Here's how the part is built. I have some questions about the finished solid (model axes, mm). A direction names the side the tool comes from. Give positions to 0.01 mm unless a question says otherwise; leave off trailing zeros. Loops run counter-clockwise (first coordinate to the right, second up) from the corner with the lowest first, then second, coordinate; pieces in that order, holes last. Notation, with made-up numbers: (68, 35) - (117, 35) arc R27 ccw to (117, 66) - close; hole circle Ø3 at (2.5, 77). An arc over 180 degrees is marked (long way). One line per item, written item: value. Start each with the question number.
```python
from build123d import *

# Parameters (mm, degrees)
F1_DEPTH = 2.54
F2_SIZE  = 2.53999
F4_DEPTH = 2.54
F5_SIZE  = 2.032


# Not quite as in the source:
# - a fillet or chamfer is up to 0.001 mm smaller than in the source, because OpenCascade refuses the exact size


with BuildPart() as f1:
    # F0 (on Top) → F1 (new body, symmetric)
    with BuildSketch(Plane.XY):
        Polygon((14.4337567297, -25), (14.4337567297, 25), (-28.8675134595, 0), align=None)
    extrude(amount=F1_DEPTH, both=True)

    # F2 (size 2.54 in the source; OpenCascade refuses exactly that, so slightly less here)
    f2_edges = [f1.edges().sort_by_distance(p)[0] for p in [
        (-7.216878, 12.5, 2.54),
        (-7.216878, -12.5, 2.54),
        (-7.216878, -12.5, -2.54),
        (-7.216878, 12.5, -2.54),
    ]]
    chamfer(f2_edges, length=F2_SIZE)

    # F3 (on Front) → F4 (join, symmetric)
    with BuildSketch(Plane.XZ):
        Polygon((14.3245235085, -24.810802511), (14.3245235085, 24.810802511), (-28.6490470171, 0), align=None)
    extrude(amount=F4_DEPTH, both=True)

    # F5
    f5_edges = [f1.edges().sort_by_distance(p)[0] for p in [
        (-7.162262, 2.54, 12.405401),
        (-7.162262, -2.54, 12.405401),
        (-7.162262, -2.54, -12.405401),
        (-7.162262, 2.54, -12.405401),
    ]]
    chamfer(f5_edges, length=F5_SIZE)


solid = f1.part
```
(1) For faces 1 (the face through (14.325, 0, -14)), 2 (the face through (14.325, 0, 14)), 3 (the face through (-4.646, -12.498, -1.288)), which set-ups out of +Z, -Z, +X, -X, +Y, -Y let a thin tool reach every point of the face, with its end or its side?
(2) If we section it at B-B on z = -17.5: List the corners of the cut face in (x, y) for me.
(3) Please list where these lines run through material, in increasing order: probe 1 along Z at (x, y) = (-7.5, -7.5); probe 2 along Y at (x, z) = (-11, -0.5). Write a range as from..to.
(4) Will these pins go through, and if not, where does the flat tip stop? pin 1 (5 mm diameter, centred on y = 3.5, z = 19.5, fed in from +X); pin 2 (10 mm diameter, centred on x = -2, y = 2, fed in from -Z); pin 3 (2 mm diameter, centred on x = 9, y = 16, fed in from -Z); pin 4 (4 mm diameter, centred on x = -19, z = 8, fed in from +Y).
Found:
1. face 1: -Z, +X, +Y, -Y
1. face 2: +Z, +X, +Y, -Y
1. face 3: -Z, -X, -Y
2. outline: (1.66, -0.51) - (5.73, -2.54) - (14.32, -2.54) - (14.32, 2.54) - (5.73, 2.54) - (1.66, 0.51) - close
3. probe 1: -2.54..2.54
3. probe 2: -9.74..9.74
4. pin 1: x = 14.32
4. pin 2: z = -18.14
4. pin 3: z = -2.54
4. pin 4: through
